The listing builds one solid part. Answer for the finished solid, in the listing's coordinates (mm). Face numbers are marked on the shaded views. A direction names the side the tool comes from. Give positions to 0.01 mm unless a question says otherwise; leave off trailing zeros. Write each loop counter-clockwise with the first axis right and the second up, starting at its lowest first coordinate (ties: lowest second). Pieces come first, ordered by that corner, then holes. Notation, with made-up numbers: M 45.25,49 L 68.25,49 A16 ccw 68.25,66 Z; hole C 39.25,72.5 d11. An arc over 180 degrees is marked long. Answer as a JSON object with one key per item and string values.
```python
from build123d import *

# Parameters (mm, degrees)
SKETCH1_R           = 9.5
BOSS_EXTRUDE1_DEPTH = 12
CHAMFER1_SIZE       = 2
CHAMFER2_SIZE       = 1
SKETCH2_R           = 7
CUT_EXTRUDE1_DEPTH  = 14
SKETCH3_R           = 3
CUT_EXTRUDE2_DEPTH  = 14


with BuildPart() as part:
    # Sketch1 → Boss-Extrude1 (new, symmetric)
    with BuildSketch(Plane.XY):
        Circle(SKETCH1_R)
    extrude(amount=BOSS_EXTRUDE1_DEPTH, both=True)

    # Chamfer1
    chamfer1_edges = [part.edges().sort_by_distance(p)[0] for p in [
        (-9.5, 0, 12),
    ]]
    chamfer(chamfer1_edges, length=CHAMFER1_SIZE)

    # Chamfer2
    chamfer2_edges = [part.edges().sort_by_distance(p)[0] for p in [
        (-9.5, 0, -12),
    ]]
    chamfer(chamfer2_edges, length=CHAMFER2_SIZE)

    # Sketch2 → Cut-Extrude1 (cut)
    with BuildSketch(Plane(origin=(0, 0, -12), x_dir=(-1, 0, 0), z_dir=(0, 0, -1))):
        Circle(SKETCH2_R)
    extrude(amount=-CUT_EXTRUDE1_DEPTH, mode=Mode.SUBTRACT)

    # Sketch3 → Cut-Extrude2 (cut)
    with BuildSketch(Plane(origin=(0, 0, 2), x_dir=(-1, 0, 0), z_dir=(0, 0, -1))):
        Circle(SKETCH3_R)
    extrude(amount=-CUT_EXTRUDE2_DEPTH, mode=Mode.SUBTRACT)


solid = part.part
```
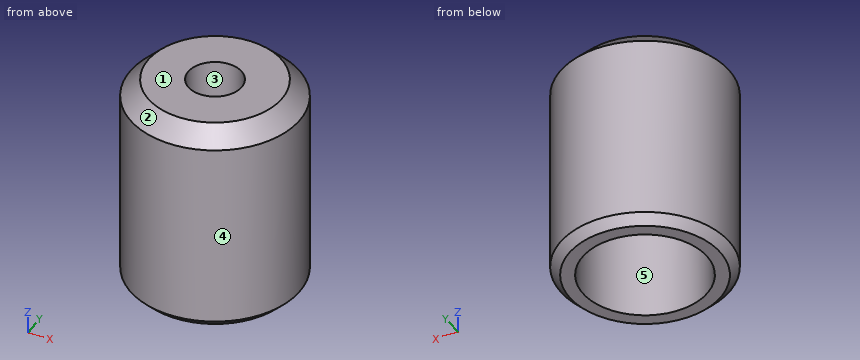
1. For the marked faces 4 and 5, determine the directions among +Z, -Z, +X, -X, +Y, -Y from which every point of the face is accessible in a straight line to the end or side of a thin tool.
Verdict:
{"face 4": "+Z, -Z", "face 5": "-Z"}
2. The mould has two halves that part along X. Classify the marked faces 1, 2 and 3: released by +X, released by -X, zero draft, split by the parting line, or undercut.
Verdict:
{"face 1": "zero draft", "face 2": "split by the parting line", "face 3": "undercut"}
3. A cutting plane is placed at C-C, the plane z = 3.5. Give the vertices of the cut face in (x, y).
Verdict:
{"outline": "C 0,0 d19; hole C 0,0 d6"}
4. Consider line 1 along Y through (x, z) = (0, -8); line 2 along Y through (x, z) = (0, 6); line 3 along X through (y, z) = (2, 8). Determine where each line is inside the solid, lowest interval first.
Verdict:
{"line 1": "y = -9.5 to -7, 7 to 9.5", "line 2": "y = -9.5 to -3, 3 to 9.5", "line 3": "x = -9.29 to -2.24, 2.24 to 9.29"}
5. A cutting plane is placed at D-D, the plane z = -3. Give the vertices of the cut face in (x, y), plus the area to 3 significant figures.
Verdict:
{"outline": "C 0,0 d19; hole C 0,0 d14", "area": "130 mm2"}
6. A cutting plane is placed at A-A, the plane x = 0. Give the vertices of the cut face in (y, z).
Verdict:
{"outline": "M -9.5,-11 L -8.5,-12 L -7,-12 L -7,2 L -3,2 L -3,12 L -7.5,12 L -9.5,10 Z; M 3,2 L 7,2 L 7,-12 L 8.5,-12 L 9.5,-11 L 9.5,10 L 7.5,12 L 3,12 Z"}
7. Flat-ended cylindrical pins translate along their axes: pin 1 (1.5 mm diameter, centred on x = -3.5, z = -3.5, fed in from -Y); pin 2 (6 mm diameter, centred on x = -5.5, z = -9.5, fed in from -Y); pin 3 (1.5 mm diameter, centred on x = -4, z = 9, fed in from +Y). Find the tip coordinate at first contact, or state that the pin passes through.
Verdict:
{"pin 1": "stops at y = -9.09", "pin 2": "stops at y = -9.17", "pin 3": "stops at y = 8.93"}
